Source: CAD feature listing. Evaluate the final solid. Frame: model axes, mm. Face numbers are marked on the shaded views. A direction names the side the tool comes from. Give positions to 0.01 mm unless a question says otherwise; leave off trailing zeros. Order: outer loops, then holes, each group sorted by start corner. A loop starts at its lowest first (then second) coordinate and runs counter-clockwise, first axis right, second up.
from build123d import *

# Parameters (mm, degrees)
BOSS_EXTRUDE1_DEPTH = 2.4


with BuildPart() as part:
    # Sketch1 → Boss-Extrude1 (new body)
    with BuildSketch(Plane(origin=(0, 0, 0), x_dir=(1, 0, 0), z_dir=(0, 1, 0))):
        with BuildLine():
            Line((3.761980861, -1.5), (3.761980861, 1.5))
            ThreePointArc((3.761980861, 1.5), (0, 4.05), (-3.761980861, 1.5))
            Line((-3.761980861, 1.5), (-3.761980861, -1.5))
            ThreePointArc((-3.761980861, -1.5), (0, -4.05), (3.761980861, -1.5))
        make_face()
    extrude(amount=BOSS_EXTRUDE1_DEPTH)

    # Sketch3 → Revolve1 (revolve)
    with BuildSketch(Plane(origin=(0, 0, 0), x_dir=(0, 0, -1), z_dir=(1, 0, 0))):
        with BuildLine():
            Line((0, 2.4), (0, 5.1))
            ThreePointArc((0, 5.1), (1.909188309, 4.309188309), (2.7, 2.4))
            Line((2.7, 2.4), (0, 2.4))
        make_face()
    revolve(axis=Axis((0, 2.4, 0), (0, 1, 0)))


solid = part.part
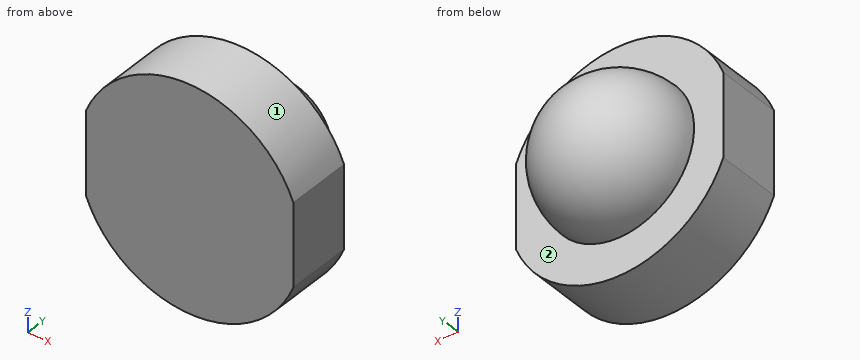
1) Section query D-D on y = 3.65. Output: boundary loops of the cut face in (x, z), and give its area (3 significant figures).
Checks:
outline: circle Ø4.79 at (0, 0)
area: 18.0 mm2
2) Ray query, L1, parallel to Y at x = 2.5, z = 2.5; L2, parallel to Y at x = -2, z = 0.75; L3, parallel to Z at x = -1.75, y = 2.7. Return the intervals inside material, ascending.
Checks:
L1: y = 0 to 2.4
L2: y = 0 to 4.05
L3: z = -2.03 to 2.03
3) Section query B-B on y = 0.5. Output: boundary loops of the cut face in (x, z), and give its area (3 significant figures).
Checks:
outline: (-3.76, -1.5) arc R4.05 ccw to (3.76, -1.5) - (3.76, 1.5) arc R4.05 ccw to (-3.76, 1.5) - close
area: 50.4 mm2
4) Section query C-C on x = 1. Output: boundary loops of the cut face in (y, z).
Checks:
outline: (0, -3.92) - (2.4, -3.92) - (2.4, -2.51) arc R2.51 ccw to (2.4, 2.51) - (2.4, 3.92) - (0, 3.92) - close
5) Reachability of the marked faces 1 and 2 from +Z, -Z, +X, -X, +Y, -Y: full face, straight path, thin tool, end or side. Return the list, or none.
Checks:
face 1: +Z, +Y, -Y
face 2: +Y
6) Section query A-A on z = 1. Output: boundary loops of the cut face in (x, y).
Checks:
outline: (-3.76, 0) - (3.76, 0) - (3.76, 2.4) - (2.51, 2.4) arc R2.51 ccw to (-2.51, 2.4) - (-3.76, 2.4) - close
7) First-contact query: pin 1 Ø2 at (x, z) = (2.5, 2) entering from +Y. Flat tip, straight axial feed; report the tip coordinate or a pass-through.
Checks:
pin 1: stops at y = 3.96
